Answer from the drawing. Dimensions are ordinates in mm from the lowest x, y and z of the part. A direction names the side the tool comes from. Round coordinates to 2 decimals unless told otherwise and drop trailing zeros. Loops run counter-clockwise (first coordinate to the right, second up) from the corner with the lowest first, then second, coordinate; pieces in that order, holes last. Notation, with made-up numbers: (16, 77) - (39, 77) arc R14 ccw to (39, 83) - close; hole circle Ø1 at (-25, -3.5). An arc over 180 degrees is marked (long way). Answer as CSV lines item,"result".
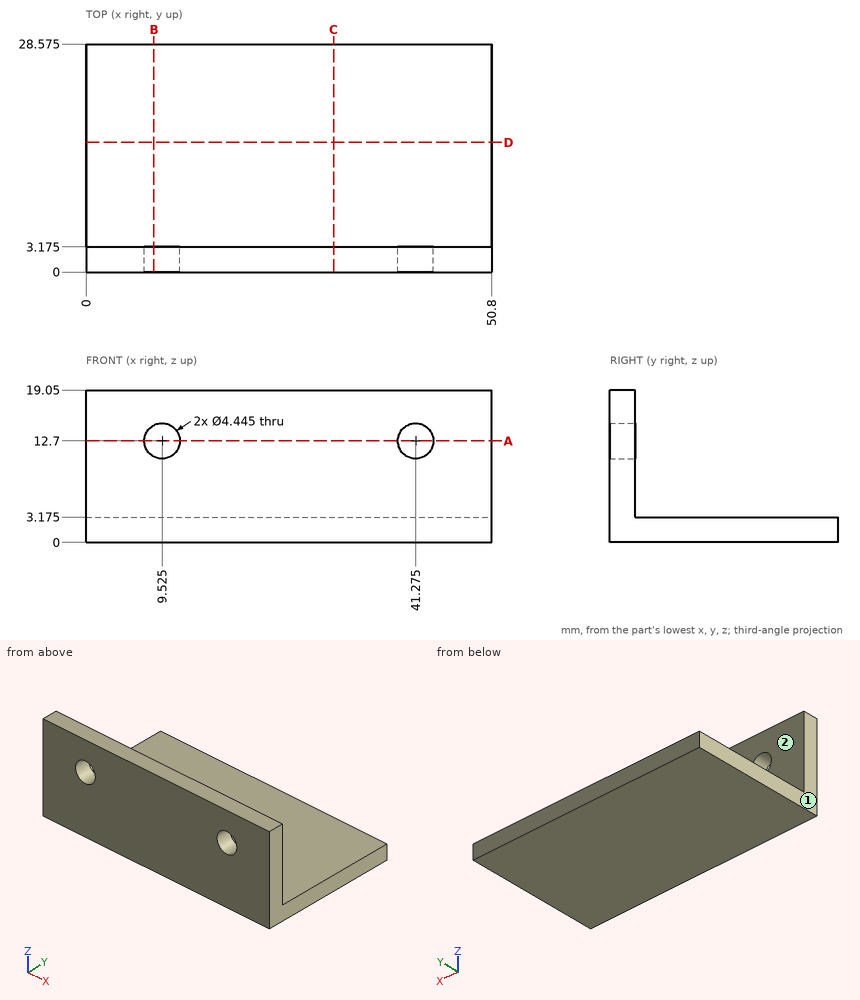
1) Find the intervals of material crossed by line 1 (Z direction, x = 7, y = 16.75) (3 decimals), in increasing order.
Entries:
line 1,"z = 0 to 3.175"
2) Each of these flat-tipped pins is pushed along its axis until it touches: P1, Ø10, axis at x = 38.5, z = 16, coming from the +Y side (3 decimals); P2, Ø4, axis at x = 21, y = 23, coming from the +Z side (3 decimals); P3, Ø2.5, axis at x = 41.275, z = 12.7, coming from the +Y side. Where does it stop, or does it pass through?
Entries:
P1,"stops at y = 3.175"
P2,"stops at z = 3.175"
P3,"passes through"
3) A tool of negligible diameter and unlimited length cuts with its end or side. For the marked faces 1 and 2, from which of +Z, -Z, +X, -X, +Y, -Y can it reach the whole face along a straight path? Write none if from no direction.
Entries:
face 1,"+Z, -Z, -X, +Y, -Y"
face 2,"+Z, +X, -X, +Y"
4) A cutting plane is placed at A-A, the plane z = 12.7. Determine the outline of the cut face in (x, y) (1 decimal), plus the area to 3 significant figures.
Entries:
outline,"(0, 0) - (7.3, 0) - (7.3, 3.2) - (0, 3.2) - close; (11.7, 0) - (39.1, 0) - (39.1, 3.2) - (11.7, 3.2) - close; (43.5, 0) - (50.8, 0) - (50.8, 3.2) - (43.5, 3.2) - close"
area,"133 mm^2"
5) A cutting plane is placed at B-B, the plane x = 8.5. Determine the outline of the cut face in (y, z) (3 decimals).
Entries:
outline,"(0, 0) - (28.575, 0) - (28.575, 3.175) - (3.175, 3.175) - (3.175, 10.728) - (0, 10.728) - close; (0, 14.672) - (3.175, 14.672) - (3.175, 19.05) - (0, 19.05) - close"
6) A cutting plane is placed at D-D, the plane y = 16.25. Determine the outline of the cut face in (x, z) (3 decimals), plus the area to 3 significant figures.
Entries:
outline,"(0, 0) - (50.8, 0) - (50.8, 3.175) - (0, 3.175) - close"
area,"161 mm^2"
7) A cutting plane is placed at C-C, the plane x = 31. Determine the outline of the cut face in (y, z) (3 decimals).
Entries:
outline,"(0, 0) - (28.575, 0) - (28.575, 3.175) - (3.175, 3.175) - (3.175, 19.05) - (0, 19.05) - close"
